Autodesk Fusion 360 part; units mm, degrees
sketch "Sketch1" plane through (0, 0, 0) normal (0, 0, 1) x (1, 0, 0)
  line L0 (8, -8) -> (-8, -8)
  line L1 (-8, -8) -> (-8, 8)
  line L2 (-8, 8) -> (8, 8)
  line L3 (8, 8) -> (8, -8)
  line L4 (8, -8) -> (-8, 8) construction
  line L5 (-8, -8) -> (8, 8) construction
  line L6 (1.525, 1) -> (-1.525, 1)
  line L7 (-1.525, 1) -> (-1.525, -1)
  line L8 (-1.525, -1) -> (1.525, -1)
  line L9 (1.525, -1) -> (1.525, 1)
  line L10 (1.525, 1) -> (-1.525, -1) construction
  line L11 (-1.525, 1) -> (1.525, -1) construction
  line L12 (1.475, 1) -> (-1.475, 1)
  line L13 (-1.475, 1) -> (-1.475, -1)
  line L14 (-1.475, -1) -> (1.475, -1)
  line L15 (1.475, -1) -> (1.475, 1)
  line L16 (1.475, 1) -> (-1.475, -1) construction
  line L17 (-1.475, 1) -> (1.475, -1) construction
  line L18 (8.6603, -5) -> (8.6603, 5)
  line L19 (8.6603, 5) -> (0, 10)
  line L20 (0, 10) -> (-8.6603, 5)
  line L21 (-8.6603, 5) -> (-8.6603, -5)
  line L22 (-8.6603, -5) -> (0, -10)
  line L23 (0, -10) -> (8.6603, -5)
  dimension "d1" = 16
  dimension "d2" = 16
  dimension "d14" = 3.05
  dimension "d15" = 2
  dimension "d16" = 2.95
  dimension "d17" = 2
  dimension "d20" = 10
extrude "Extrude1" add sketch "Sketch1" along normal blind 7 contours L0 L22 L23 | L0 L1 L2 L3 L19 L20 L22 L23 | L3 L18 L19 L23 | L1 L20 L21 L22 | L2 L19 L20 | L6 L8 L9 L15 | L6 L8 L12 L13 L14 L15 | L6 L7 L8 L13
fillet "Fillet1" radius 0.2 7 faces at (0, -3.3333, 7) (2.8868, -8.3333, 2.3333) (8.6603, -1.6667, 4.6667) (-5.7735, -6.6667, 4.6667) (-8.6603, 1.6667, 4.6667) (-2.8868, 8.3333, 2.3333) (5.7735, 6.6667, 4.6667)
extrude "Extrude4" cut sketch "Sketch1" along normal blind 2.8 contours L6 L8 L9 L15 | L6 L8 L12 L13 L14 L15 | L6 L7 L8 L13
Verification items for the finished model (mm, model axes). A direction names the side the tool comes from. Coordinates: 2 decimals unless noted, no trailing zeros. Loops run counter-clockwise (first coordinate to the right, second up) from the corner with the lowest first, then second, coordinate; pieces in that order, holes last. Notation, with made-up numbers: (48, 52) -> (53, 52) arc R17 cw to (53, 70) -> close; hole circle Ø6 at (23.5, 52). An arc over 180 degrees is marked (long way). Answer in a Markdown table with one row per item. Add a question column.
1. Depth check by flat-ended pin: P1, Ø2, axis at x = -5, z = 3, coming from the -Y side; P2, Ø0.8, axis at x = -0.5, z = 1.5, coming from the +Y side. Enter the tip coordinate at first touch or a pass-through.
2. Material ranges on probe 1 along X at (y, z) = (-0.25, 1) (3 decimals); probe 2 along Z at (x, y) = (-5.75, 6.5); probe 3 along Z at (x, y) = (0, 0.75), recorded low to high. Write a range as [from, to].
3. Access from +Z, -Z, +X, -X, +Y, -Y to the whole of each face (thin tool, end or side, straight path). Record for faces 1 (the face through (0, 0, 2.8)), 2 (the face through (-4.271, 7.534, 3.454)).
4. Section check B-B, the plane z = 0.5. Enter the section's corners in (x, y) (3 decimals).
5. Section check C-C, the plane z = 6. Enter the section's corners in (x, y).
6. Draft check along X on faces 3 (the face through (1.525, 0, 1)), 4 (the face through (-4.242, -7.485, 0.06)), 5 (the face through (4.389, 7.466, 3.454)), 6 (the face through (0, -2, 0)). Enter one of: +X half, -X half, draft (parallel to the pull), parting line (faces both ways), or undercut.
7. Section check A-A, the plane y = 0. Enter the section's corners in (x, z) (3 decimals), then the cut area to 3 significant figures.
Derived:
| question | item | result |
|---|---|---|
| 1 | P1 | stops at y = -7.69 |
| 1 | P2 | stops at y = 9.94 |
| 2 | probe 1 | x = [-8.66, -1.525], [1.525, 8.66] |
| 2 | probe 2 | z = [0, 7] |
| 2 | probe 3 | z = [2.8, 7] |
| 3 | face 1 | -Z |
| 3 | face 2 | +Z, -Z, -X, +Y |
| 4 | outline | (-8.66, -4.885) arc R0.2 ccw to (-8.56, -5.058) -> (-0.1, -9.942) arc R0.2 ccw to (0.1, -9.942) -> (8.56, -5.058) arc R0.2 ccw to (8.66, -4.885) -> (8.66, 4.885) arc R0.2 ccw to (8.56, 5.058) -> (0.1, 9.942) arc R0.2 ccw to (-0.1, 9.942) -> (-8.56, 5.058) arc R0.2 ccw to (-8.66, 4.885) -> close; hole (-1.525, -1) -> (1.525, -1) -> (1.525, 1) -> (-1.525, 1) -> close |
| 5 | outline | (-8.66, -4.88) arc R0.2 ccw to (-8.56, -5.06) -> (-0.1, -9.94) arc R0.2 ccw to (0.1, -9.94) -> (8.56, -5.06) arc R0.2 ccw to (8.66, -4.88) -> (8.66, 4.88) arc R0.2 ccw to (8.56, 5.06) -> (0.1, 9.94) arc R0.2 ccw to (-0.1, 9.94) -> (-8.56, 5.06) arc R0.2 ccw to (-8.66, 4.88) -> close |
| 6 | face 3 | undercut |
| 6 | face 4 | -X half |
| 6 | face 5 | +X half |
| 6 | face 6 | draft |
| 7 | outline | (-8.66, 0.2) arc R0.2 ccw to (-8.46, 0) -> (-1.525, 0) -> (-1.525, 2.8) -> (1.525, 2.8) -> (1.525, 0) -> (8.46, 0) arc R0.2 ccw to (8.66, 0.2) -> (8.66, 6.8) arc R0.2 ccw to (8.46, 7) -> (-8.46, 7) arc R0.2 ccw to (-8.66, 6.8) -> close |
| 7 | area | 113 mm² |
